The listing builds one solid part. Answer for the finished solid, in the listing's coordinates (mm). A direction names the side the tool comes from. Round coordinates to 2 decimals unless told otherwise and drop trailing zeros. Write each loop counter-clockwise with the first axis right and the second up, starting at its lowest first coordinate (ties: lowest second). Pieces come first, ordered by that corner, then holes.
from build123d import *

# Parameters (mm, degrees)
SKETCH1_W           = 8.6106
SKETCH1_H           = 4.3942
BOSS_EXTRUDE1_DEPTH = 7.493
SKETCH2_W           = 0.4064
SKETCH2_H           = 0.4064
CUT_EXTRUDE1_DEPTH  = 13.230963781
CUT_EXTRUDE4_DEPTH  = 7.0866
FILLET8_R           = 0.381
CUT_EXTRUDE5_DEPTH  = 13.230963781
CUT_EXTRUDE6_DEPTH  = 13.230963781
BOSS_EXTRUDE2_DEPTH = 0.396875
SKETCH7_W           = 0.396875
SKETCH7_H           = 0.3937
BOSS_EXTRUDE3_DEPTH = 0.396875
SKETCH8_W           = 0.396875
SKETCH8_H           = 0.396875
BOSS_EXTRUDE4_DEPTH = 0.396875
FILLET9_R           = 0.381
FILLET10_R          = 0.0508
CUT_EXTRUDE7_REACH  = 14.231
SKETCH9_W           = 4.1148
SKETCH9_H           = 2.1082
SKETCH11_W          = 2.0066
SKETCH11_H          = 2.0066
BOSS_EXTRUDE5_DEPTH = 4.384675
SKETCH12_W          = 4.487424853
SKETCH12_H          = 2.672562517
BOSS_EXTRUDE6_DEPTH = 1.5748
CUT_EXTRUDE10_REACH = 13.587
SKETCH14_W          = 0.508
SKETCH14_H          = 0.3048
BOSS_EXTRUDE7_DEPTH = 3.048
FILLET11_R          = 0.2413


with BuildPart() as part:
    # Sketch1 → Boss-Extrude1 (new body)
    with BuildSketch(Plane(origin=(0, 0, 0), x_dir=(1, 0, 0), z_dir=(0, 1, 0))):
        with Locations((4.3053, 2.1971)):
            Rectangle(SKETCH1_W, SKETCH1_H)
    extrude(amount=-BOSS_EXTRUDE1_DEPTH)

    # Sketch2 → Cut-Extrude1 (cut, through all)
    with BuildSketch(Plane(origin=(0, 0, 0), x_dir=(1, 0, 0), z_dir=(0, 1, 0))):
        with Locations((8.4074, 4.191)):
            Rectangle(SKETCH2_W, SKETCH2_H)
        with Locations((0.2032, 4.191)):
            Rectangle(SKETCH2_W, SKETCH2_H)
        with Locations((8.4074, 0.2032)):
            Rectangle(SKETCH2_W, SKETCH2_H)
        with Locations((0.2032, 0.2032)):
            Rectangle(SKETCH2_W, SKETCH2_H)
    extrude(amount=-CUT_EXTRUDE1_DEPTH, mode=Mode.SUBTRACT)

    # Sketch3 → Cut-Extrude4 (cut)
    with BuildSketch(Plane.XZ.offset(7.493)):
        with BuildLine():
            Line((0.4191, -0.4064), (8.1915, -0.4064))
            ThreePointArc((8.1915, -0.4064), (8.213180256, -0.397419744), (8.2042, -0.4191))
            Line((8.2042, -0.4191), (8.2042, -3.9751))
            ThreePointArc((8.2042, -3.9751), (8.213180256, -3.996780256), (8.1915, -3.9878))
            Line((8.1915, -3.9878), (0.4191, -3.9878))
            ThreePointArc((0.4191, -3.9878), (0.397419744, -3.996780256), (0.4064, -3.9751))
            Line((0.4064, -3.9751), (0.4064, -0.4191))
            ThreePointArc((0.4064, -0.4191), (0.397419744, -0.397419744), (0.4191, -0.4064))
        make_face()
    extrude(amount=-CUT_EXTRUDE4_DEPTH, mode=Mode.SUBTRACT)

    # Fillet8
    fillet8_edges = [part.edges().sort_by_distance(p)[0] for p in [
        (0, 0, -2.1971),
        (4.3053, 0, -4.3942),
        (8.6106, 0, -2.1971),
        (4.3053, 0, 0),
    ]]
    fillet(fillet8_edges, radius=FILLET8_R)

    # Sketch4 → Cut-Extrude5 (cut, through all)
    with BuildSketch(Plane.XY):
        Polygon((1.20015, -3.9116), (7.41045, -3.9116), (7.41045, -4.699), (7.807325, -4.699), (7.807325, -4.302125), (8.2042, -4.302125), (8.2042, -7.493), (0.4064, -7.493), (0.4064, -4.302125), (0.803275, -4.302125), (0.803275, -4.699), (1.20015, -4.699), align=None)
    extrude(amount=-CUT_EXTRUDE5_DEPTH, mode=Mode.SUBTRACT)

    # Sketch5 → Cut-Extrude6 (cut, through all)
    with BuildSketch(Plane(origin=(8.6106, 0, 0), x_dir=(0, 0, -1), z_dir=(1, 0, 0))):
        with BuildLine():
            Line((0.4064, -4.699), (1.1938, -4.699))
            ThreePointArc((1.1938, -4.699), (1.616523828, -4.330724179), (1.923404732, -4.799922032))
            Line((1.923404732, -4.799922032), (1.620182585, -5.875006123))
            ThreePointArc((1.620182585, -5.875006123), (1.600211037, -6.016040651), (1.61836436, -6.157320719))
            Line((1.61836436, -6.157320719), (1.91945657, -7.280006107))
            ThreePointArc((1.91945657, -7.280006107), (2.022134094, -7.433618006), (2.1971, -7.493))
            ThreePointArc((2.1971, -7.493), (2.372065906, -7.433618006), (2.47474343, -7.280006107))
            Line((2.47474343, -7.280006107), (2.77583564, -6.157320719))
            ThreePointArc((2.77583564, -6.157320719), (2.793988963, -6.016040651), (2.774017415, -5.875006123))
            Line((2.774017415, -5.875006123), (2.470795268, -4.799922032))
            ThreePointArc((2.470795268, -4.799922032), (2.777676172, -4.330724179), (3.2004, -4.699))
            Line((3.2004, -4.699), (3.9878, -4.699))
            Line((3.9878, -4.699), (3.9878, -7.640446321))
            Line((3.9878, -7.640446321), (0.4064, -7.640446321))
            Line((0.4064, -7.640446321), (0.4064, -4.699))
        make_face()
    extrude(amount=-CUT_EXTRUDE6_DEPTH, mode=Mode.SUBTRACT)



with BuildPart() as body_2:
    # Sketch6 → Boss-Extrude2 (new body)
    with BuildSketch(Plane.XZ.offset(3.9116)):
        Polygon((0.455456934, -0.567114284), (1.251351798, -0.567114284), (1.251351798, -0.041523335), (7.355715241, -0.041523335), (7.355715241, -0.567114284), (8.159118548, -0.567114284), (8.159118548, -3.810761279), (7.355715241, -3.810761279), (7.355715241, -4.351369112), (1.251351798, -4.351369112), (1.251351798, -3.810761279), (0.455456934, -3.810761279), align=None)
    extrude(amount=BOSS_EXTRUDE2_DEPTH)


with BuildPart() as part_1:
    add(part.part)

    add(body_2.part)  # Boss-Extrude3 merges body 2
    # Sketch7 → Boss-Extrude3 (add)
    with BuildSketch(Plane(origin=(0, 0, -0.4064), x_dir=(-1, 0, 0), z_dir=(0, 0, -1))):
        with Locations((-1.0017125, -4.50215)):
            Rectangle(SKETCH7_W, SKETCH7_H)
        with Locations((-7.6088875, -4.50215)):
            Rectangle(SKETCH7_W, SKETCH7_H)
    extrude(amount=BOSS_EXTRUDE3_DEPTH)

    # Sketch8 → Boss-Extrude4 (add)
    with BuildSketch(Plane.XY.offset(-3.9878)):
        with Locations((1.0017125, -4.5005625)):
            Rectangle(SKETCH8_W, SKETCH8_H)
        with Locations((7.6088875, -4.5005625)):
            Rectangle(SKETCH8_W, SKETCH8_H)
    extrude(amount=BOSS_EXTRUDE4_DEPTH)

    # Fillet9
    fillet9_edges = [part_1.edges().sort_by_distance(p)[0] for p in [
        (7.6088875, -4.699, -4.3942),
        (1.0017125, -4.699, -4.3942),
        (1.0017125, -4.699, 0),
        (7.6088875, -4.699, 0),
    ]]
    fillet(fillet9_edges, radius=FILLET9_R)

    # Fillet10
    # the kernel refuses this fillet: 0.0508 mm, written as the material it adds along each edge
    with BuildSketch(Plane(origin=(1.20015, -4.3053, -0.4064), x_dir=(0, 1, 0), z_dir=(-1, 0, 0)), Plane(origin=(0.803275, -4.302125, -3.9878), x_dir=(0, 1, 0), z_dir=(1, 0, 0))) as fillet10_piece_1:
        with BuildLine():
            CenterArc((FILLET10_R, FILLET10_R), FILLET10_R, 180, 90)
            Line((0, FILLET10_R), (0, 0))
            Line((0, 0), (FILLET10_R, 0))
        make_face()
    extrude(amount=0.396875)
    with BuildSketch(Plane(origin=(7.41045, -4.3053, -0.4064), x_dir=(0, 1, 0), z_dir=(1, 0, 0)), Plane(origin=(7.807325, -4.302125, -3.9878), x_dir=(0, 1, 0), z_dir=(-1, 0, 0))) as fillet10_piece_2:
        with BuildLine():
            CenterArc((FILLET10_R, -FILLET10_R), FILLET10_R, 90, 90)
            Line((0, -FILLET10_R), (0, 0))
            Line((0, 0), (FILLET10_R, 0))
        make_face()
    extrude(amount=0.396875)

    # Sketch9 → Cut-Extrude7 (cut, up to next)
    with BuildSketch(Plane.XY, mode=Mode.PRIVATE) as cut_extrude7_sk1:
        with Locations((4.3053, -2.1082)):
            Rectangle(SKETCH9_W, SKETCH9_H)
    cut_extrude7_tool1 = extrude(cut_extrude7_sk1.sketch, amount=-CUT_EXTRUDE7_REACH, mode=Mode.PRIVATE) & part_1.part
    add(cut_extrude7_tool1.solids().sort_by_distance((4.3053, -2.1082, 0))[0], mode=Mode.SUBTRACT)



with BuildPart() as body_2_2:
    # Sketch11 → Boss-Extrude5 (new body)
    with BuildSketch(Plane(origin=(0, 0, -0.4064), x_dir=(-1, 0, 0), z_dir=(0, 0, -1))):
        with Locations((-3.349764598, -2.1082)):
            Rectangle(SKETCH11_W, SKETCH11_H)
    extrude(amount=-BOSS_EXTRUDE5_DEPTH)


with BuildPart() as part_2:
    add(part_1.part)

    add(body_2_2.part)  # Boss-Extrude6 merges body 2 2
    # Sketch12 → Boss-Extrude6 (add)
    with BuildSketch(Plane(origin=(0, 0, -0.4064), x_dir=(-1, 0, 0), z_dir=(0, 0, -1))):
        with Locations((-4.248970079, -2.082014044)):
            Rectangle(SKETCH12_W, SKETCH12_H)
    extrude(amount=BOSS_EXTRUDE6_DEPTH)

    # Sketch13 → Cut-Extrude10 (cut, up to next)
    with BuildSketch(Plane(origin=(0, -1.1049, 0), x_dir=(1, 0, 0), z_dir=(0, 1, 0)), mode=Mode.PRIVATE) as cut_extrude10_sk1:
        Polygon((2.968764598, -3.978275), (3.349764598, -3.597275), (3.730764598, -3.978275), align=None)
    cut_extrude10_tool1 = extrude(cut_extrude10_sk1.sketch, amount=-CUT_EXTRUDE10_REACH, mode=Mode.PRIVATE) & part_2.part
    add(cut_extrude10_tool1.solids().sort_by_distance((3.349765, -1.1049, 3.851275))[0], mode=Mode.SUBTRACT)

    # Sketch14 → Boss-Extrude7 (add)
    with BuildSketch(Plane.XZ.offset(4.308475)):
        with Locations((6.3119, -2.1971)):
            Rectangle(SKETCH14_W, SKETCH14_H)
        with Locations((2.2987, -2.1971)):
            Rectangle(SKETCH14_W, SKETCH14_H)
        with Locations((4.3053, -2.1971)):
            Rectangle(SKETCH14_W, SKETCH14_H)
    extrude(amount=BOSS_EXTRUDE7_DEPTH)

    # Fillet11
    fillet11_edges = [part_2.edges().sort_by_distance(p)[0] for p in [
        (6.5659, -7.356475, -2.1971),
        (6.0579, -7.356475, -2.1971),
        (2.5527, -7.356475, -2.1971),
        (2.0447, -7.356475, -2.1971),
        (4.5593, -7.356475, -2.1971),
        (4.0513, -7.356475, -2.1971),
    ]]
    fillet(fillet11_edges, radius=FILLET11_R)


solid = part_2.part
1. Given pin 1 (2 mm diameter, centred on y = -1.5, z = 2.5, fed in from +X), flat-ended and moving along its own axis, determine where the tip first touches the part or whether it passes through.
Geometry says:
pin 1: stops at x = 4.35
2. Section D-D on x = 2.75 is taken. Determine the outline of the cut face in (y, z).
Geometry says:
outline: (-4.31, -4.35) - (-3.91, -4.35) - (-3.91, -4.39) - (-0.38, -4.39) arc R0.38 ccw to (0, -4.01) - (0, -0.38) arc R0.38 ccw to (-0.38, 0) - (-1.05, 0) - (-1.05, -0.41) - (-1.1, -0.41) - (-1.1, 3.98) - (-3.11, 3.98) - (-3.11, -0.41) - (-3.16, -0.41) - (-3.16, 0) - (-3.91, 0) - (-3.91, -0.04) - (-4.31, -0.04) - close; hole (-3.91, -3.99) - (-0.41, -3.99) - (-0.41, -0.41) - (-0.75, -0.41) - (-0.75, -1.98) - (-3.42, -1.98) - (-3.42, -0.41) - (-3.91, -0.41) - close
3. Straight lines are drawn through the part: line 1 along Y through (x, z) = (6.25, -1); line 2 along Z through (x, y) = (5.75, -3.75); line 3 along Y through (x, z) = (4.75, -3.5). For each, find the intervals that lie inside material, in ascending order.
Geometry says:
line 1: y = -4.31 to -3.91, -3.42 to -0.75, -0.41 to 0
line 2: z = -4.39 to -3.99, -0.41 to 0
line 3: y = -4.31 to -3.91, -0.41 to 0
4. Section A-A on x = 7 is taken. Determine the outline of the cut face in (y, z).
Geometry says:
outline: (-4.31, -4.35) - (-3.91, -4.35) - (-3.91, -4.39) - (-0.38, -4.39) arc R0.38 ccw to (0, -4.01) - (0, -0.38) arc R0.38 ccw to (-0.38, 0) - (-3.91, 0) - (-3.91, -0.04) - (-4.31, -0.04) - close; hole (-3.91, -3.99) - (-0.41, -3.99) - (-0.41, -0.41) - (-3.91, -0.41) - close
5. A tool of negligible diameter and unlimited length cuts with its end or side. For faces 4 (the face through (4.3, -3.7, -0.406)), 5 (the face through (8.611, -3, -2)), from which of +Z, -Z, +X, -X, +Y, -Y can it reach the whole face along a straight path? Write none if from no direction.
Geometry says:
face 4: none
face 5: +Z, -Z, +X, +Y, -Y
6. For a pull along Y with two mould halves and no side action, classify faces 1 (the face through (0.406, -3, -2)), 2 (the face through (4, 0, -2)), 3 (the face through (4, -0.746, -1)) as released by +Y, released by -Y, zero draft, split by the parting line, or undercut.
Geometry says:
face 1: zero draft
face 2: released by +Y
face 3: undercut
7. Section C-C on y = -2 is taken. Give the number of separate pieces and of enclosed holes in the cut face, plus the area to 3 significant figures.
Geometry says:
separate pieces: 4
enclosed holes: 0
area: 23.3 mm2
8. Section B-B on y = -5.5 is taken. Determine the outline of the cut face in (x, z).
Geometry says:
outline: (0, -2.67) - (0.41, -2.67) - (0.41, -1.73) - (0, -1.73) - close; (2.04, -2.35) - (2.55, -2.35) - (2.55, -2.04) - (2.04, -2.04) - close; (4.05, -2.35) - (4.56, -2.35) - (4.56, -2.04) - (4.05, -2.04) - close; (6.06, -2.35) - (6.57, -2.35) - (6.57, -2.04) - (6.06, -2.04) - close; (8.2, -2.67) - (8.61, -2.67) - (8.61, -1.73) - (8.2, -1.73) - close
